Build history of the part. All positions in model axes, mm. A direction names the side the tool comes from. Give positions to 0.01 mm unless a question says otherwise; leave off trailing zeros. Order: outer loops, then holes, each group sorted by start corner. A loop starts at its lowest first (then second) coordinate and runs counter-clockwise, first axis right, second up. Notation, with made-up numbers: (-2.5, -17.75) -> (9.5, -17.75) arc R25 cw to (9.5, 21.25) -> close; hole circle Ø6 at (82.5, 35.5). An arc over 180 degrees is marked (long way). One line per question, with ' | ' between items. Start each with the question number.
(1) Pull direction Z, two halves, no side cores. Call faces 5 (the face through (-20.4, -20.43, 15.49)), 6 (the face through (-1.3, -1.1, 24)), 7 (the face through (0, 0, 30)), 8 (the face through (-1.5, -0.07, 19.94)): +Z half, -Z half, draft (parallel to the pull), parting line (faces both ways), or undercut.
(2) Cut at A-A (x = -4). Give the cut face in (y, z), then the cut area to 3 significant figures.
(3) Cut at D-D (x = 11). Give the cut face in (y, z), then the cut area to 3 significant figures.
(4) Drill centre lines: L1, parallel to Z at x = -3, y = 1; L2, parallel to Z at x = 9, y = -4; L3, parallel to Y at x = -4, z = 13. Where is each one in solid material? Low to high. Write a range as from..to.
(5) Cut at B-B (y = -3.5). Give the cut face in (x, z), then the cut area to 3 significant figures.
(6) Pin check, flat tips, straight feed: pin 1 Ø12 at (x, y) = (16, 12.5) entering from +Z; pin 2 Ø8 at (x, z) = (5.5, 11) entering from -Y; pin 3 Ø4 at (y, z) = (3.5, 9) entering from -X. Stop position of each tip, or through.
(7) Which spindle directions (+Z, -Z, +X, -X, +Y, -Y) get a long thin tool onto all of the face, cutting with end or side? Do faces 1 (the face through (16, 17, 15)), 2 (the face through (-1.19, -5.37, 27.04)), 3 (the face through (-16, -16, 15)), 4 (the face through (20.03, -6.31, 7.89)). Say none if no direction does.
(8) Cut at C-C (z = 21.5). Give the cut face in (x, y).
Autodesk Inventor part; units mm, degrees
ref_plane "YZ Plane" through (0, 0, 0) normal (1, 0, 0) x (0, 1, 0)
ref_plane "XZ Plane" through (0, 0, 0) normal (0, 1, 0) x (-1, 0, 0)
ref_plane "XY Plane" through (0, 0, 0) normal (0, 0, 1) x (1, 0, 0)
sketch "Sketch1" plane through (0, 0, 0) normal (0, 0, 1) x (1, 0, 0)
  circle A0 centre (0, 0) radius 21
  dimension "d0" = 42
extrude "Extrusion1" add sketch "Sketch1" along normal blind 15
sketch "Sketch2" plane through (0, 0, 15) normal (0, 0, 1) x (1, 0, 0)
  circle A0 centre (0, 0) radius 21 construction
  circle A1 centre (0, 0) radius 1.5
  dimension "d3" = 3
extrude "Extrusion2" add sketch "Sketch2" along normal blind 15
sketch "Sketch3" plane through (0, 0, 15) normal (0, 0, 1) x (1, 0, 0)
  circle A0 centre (0, 0) radius 1.5 construction
  circle A1 centre (0, 0) radius 21 construction
  line L0 (-19, -21) -> (0, -21)
  line L1 (21, 0) -> (21, 19)
  line L2 (19, 21) -> (0, 21)
  line L3 (-21, 0) -> (-21, -19)
  line L4 (-21, -21) -> (21, 21) construction
  line L5 (21, -21) -> (-21, 21) construction
  circle A2 centre (0, 0) radius 21
  arc A3 (21, 19) -> (19, 21) centre (19, 19) ccw
  arc A4 (-21, -19) -> (-19, -21) centre (-19, -19) ccw
  circle A5 centre (-17.6777, -17.6777) radius 1.5
  circle A6 centre (17.6777, 17.6777) radius 1.5
  point P0 (0, 0)
  dimension "d6" = 2
  dimension "d7" = 3
  dimension "d8" = 3
  dimension "d9" = 25
  dimension "d10" = 25
extrude "Extrusion3" add sketch "Sketch3" along normal blind 1
sketch "Sketch4" plane through (0, 0, 30) normal (0, 0, 1) x (1, 0, 0)
  circle A0 centre (0, 0) radius 5.5
  dimension "d13" = 11
extrude "Extrusion4" add sketch "Sketch4" against normal blind 6
properties part number "stepper motor 1"
Result set:
1) face 5: draft | face 6: undercut | face 7: +Z half | face 8: undercut
2) outline: (-21, 15) -> (-20.62, 15) -> (-20.62, 0) -> (20.62, 0) -> (20.62, 16) -> (-21, 16) -> close; (-3.77, 24) -> (3.77, 24) -> (3.77, 30) -> (-3.77, 30) -> close | area: 705 mm2
3) outline: (-17.89, 0) -> (17.89, 0) -> (17.89, 15) -> (21, 15) -> (21, 16) -> (-17.89, 16) -> close | area: 576 mm2
4) L1: z = 0..16, 24..30 | L2: z = 0..16 | L3: y = -20.62..20.62
5) outline: (-21, 15) -> (-20.71, 15) -> (-20.71, 0) -> (20.71, 0) -> (20.71, 16) -> (-21, 16) -> close; (-4.24, 24) -> (4.24, 24) -> (4.24, 30) -> (-4.24, 30) -> close | area: 714 mm2
6) pin 1: stops at z = 16 | pin 2: stops at y = -20.95 | pin 3: stops at x = -20.95
7) face 1: -Z, +X, +Y | face 2: +Z | face 3: -Z, -X, -Y | face 4: -Z
8) outline: circle Ø3 at (0, 0)
